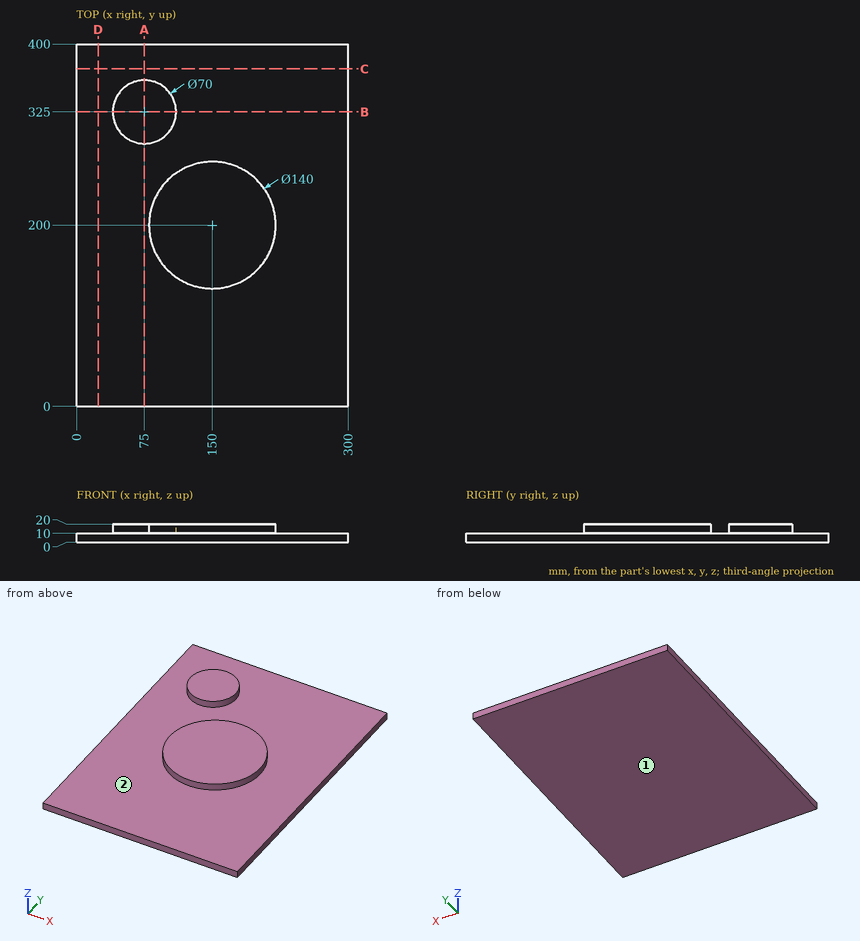
Could you check a few things on this drawing? It's one solid part, dimensions in mm from its lowest x, y, z. A direction names the side the tool comes from. Give positions to 0.01 mm unless a question says otherwise; leave off trailing zeros. Order: outer loops, then holes, each group sorted by start corner. A loop starts at its lowest first (then second) coordinate and runs counter-clockwise, first axis right, second up. Notation, with made-up numbers: M -3,50 L 34,50 A18 ccw 34,62 Z; hole C -2,-10 d8. An arc over 180 degrees is marked long. Use one line per item in the form item = value.
Item 1: If we section it at A-A, the plane x = 75: Write out the boundary of the cut face in (y, z).
Values follow:
outline = M 0,0 L 400,0 L 400,10 L 360,10 L 360,20 L 290,20 L 290,10 L 0,10 Z
Item 2: If we section it at B-B, the plane y = 325: Write out the boundary of the cut face in (x, z).
Values follow:
outline = M 0,0 L 300,0 L 300,10 L 110,10 L 110,20 L 40,20 L 40,10 L 0,10 Z
Item 3: If I drill on line 1 along Z through (x, y) = (31, 286.5); line 2 along X through (y, z) = (234, 12.25); line 3 along X through (y, z) = (168, 15.75), over which ranges is the centre line in solid material (lowest first)? Write a range as [from, to].
Values follow:
line_1 = [0, 10]
line_2 = [88.81, 211.19]
line_3 = [87.74, 212.26]
Item 4: Will these pins go through, and if not, where does the flat tip stop? pin 1 Ø12 at (x, y) = (85, 133.5) entering from -Z; pin 2 Ø2 at (x, z) = (170.5, 14) entering from +Y.
Values follow:
pin_1 = 0
pin_2 = 267.23
Item 5: If we section it at C-C, the plane y = 372.5: Write out the boundary of the cut face in (x, z), and give its area (3 significant figures).
Values follow:
outline = M 0,0 L 300,0 L 300,10 L 0,10 Z
area = 3,000 mm^2
Item 6: If we section it at D-D, the plane x = 24: Write out the boundary of the cut face in (y, z), and give its area (3 significant figures).
Values follow:
outline = M 0,0 L 400,0 L 400,10 L 0,10 Z
area = 4,000 mm^2
Item 7: For the marked faces 1 and 2, which set-ups out of +Z, -Z, +X, -X, +Y, -Y let a thin tool reach every point of the face, with its end or its side?
Values follow:
face_1 = -Z, +X, -X, +Y, -Y
face_2 = +Z
